Here's the drawing with two shaded views (mm, measured from the low corner). I have some questions. Give positions to 0.01 mm unless a question says otherwise; leave off trailing zeros. Loops run counter-clockwise (first coordinate to the right, second up) from the corner with the lowest first, then second, coordinate; pieces in that order, holes last. Notation, with made-up numbers: (-29, 29) -> (10, 29) arc R36 ccw to (10, 64) -> close; hole circle Ø9 at (39, -22.5). An arc over 180 degrees is marked (long way). Write each question's results on one line, items separated by ' | '. Start each with the question number.
Q1. If we section it at B-B, the plane x = 22.1: List the corners of the cut face in (y, z) for me.
Q2. Will this pin go through, and if not, where does the flat tip stop? P1, Ø1.2, axis at x = 22.1, y = 21.2, coming from the +Z side.
Q3. If I drill on line 1 along Y through (x, z) = (22.1, 1.45); line 2 along Y through (x, z) = (52, 1.8); line 3 along X through (y, z) = (4.5, 0.75), over which ranges is the centre line in solid material (lowest first)?
Q4. If we section it at A-A, the plane y = 21.2: List the corners of the cut face in (x, z) for me, plus the area to 3 significant figures.
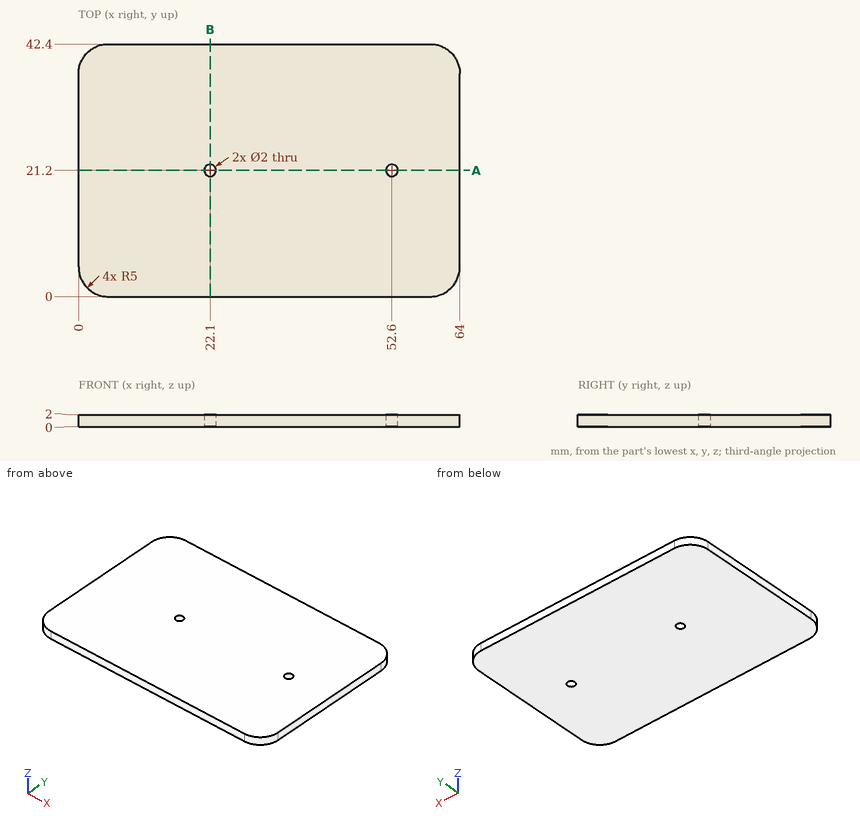
Final values:
1) outline: (0, 0) -> (20.2, 0) -> (20.2, 2) -> (0, 2) -> close; (22.2, 0) -> (42.4, 0) -> (42.4, 2) -> (22.2, 2) -> close
2) P1: passes through
3) line 1: y = 0 to 20.2, 22.2 to 42.4 | line 2: y = 0 to 20.4, 22 to 42.4 | line 3: x = 0.03 to 63.97
4) outline: (0, 0) -> (21.1, 0) -> (21.1, 2) -> (0, 2) -> close; (23.1, 0) -> (51.6, 0) -> (51.6, 2) -> (23.1, 2) -> close; (53.6, 0) -> (64, 0) -> (64, 2) -> (53.6, 2) -> close | area: 120 mm²
